```python
from build123d import *

# Parameters (mm, degrees)
SKETCH1_R           = 12.8
BOSS_EXTRUDE1_DEPTH = 23
SKETCH2_R           = 2
CUT_EXTRUDE1_DEPTH  = 7.5


with BuildPart() as part:
    # Sketch1 → Boss-Extrude1 (new, symmetric)
    with BuildSketch(Plane.XY):
        with BuildLine():
            Line((-13, -21.319), (13, -21.319))
            ThreePointArc((13, -21.319), (15.121320344, -20.440320344), (16, -18.319))
            Line((16, -18.319), (16, 12.7))
            ThreePointArc((16, 12.7), (15.121320344, 14.821320344), (13, 15.7))
            Line((13, 15.7), (-13, 15.7))
            ThreePointArc((-13, 15.7), (-15.121320344, 14.821320344), (-16, 12.7))
            Line((-16, 12.7), (-16, -18.319))
            ThreePointArc((-16, -18.319), (-15.121320344, -20.440320344), (-13, -21.319))
        make_face()
        Circle(SKETCH1_R, mode=Mode.SUBTRACT)
    extrude(amount=BOSS_EXTRUDE1_DEPTH, both=True)

    # Sketch2 → Cut-Extrude1 (cut)
    with BuildSketch(Plane(origin=(0, -21.319, 0), x_dir=(1, 0, 0), z_dir=(0, 1, 0))):
        with Locations(Location((12, -17.5, 0), (0, 0, 60))):
            Circle(SKETCH2_R)
        with Locations(Location((-12, 17.5, 0), (0, 0, 120))):
            Circle(SKETCH2_R)
    extrude(amount=CUT_EXTRUDE1_DEPTH, mode=Mode.SUBTRACT)


solid = part.part
```
The model under review builds one solid part; all positions refer to its coordinate system, in mm. A direction names the side the tool comes from. Give positions to 0.01 mm unless a question says otherwise; leave off trailing zeros. Write each loop counter-clockwise with the first axis right and the second up, starting at its lowest first coordinate (ties: lowest second). Pieces come first, ordered by that corner, then holes.
(1) Consider section B-B, the plane y = 0. Give the boundary of the cut face in (x, z), and give its area (3 significant figures).
(2) Consider section C-C, the plane z = 13.5. Give the boundary of the cut face in (x, y).
(3) Consider section D-D, the plane x = -12. Give the boundary of the cut face in (y, z).
(4) For P1, Ø1.2, axis at x = -12, z = -16.5, coming from the -Y side, flat-tipped, find the tip position at first contact; note if it passes through.
(5) To check wall thickness, follow L1, parallel to X at y = -17.25, z = 17.5; L2, parallel to Z at x = 12, y = -18.5; L3, parallel to X at y = -15.75, z = -17.5. State the ranges of each line that lie inside material, in increasing order.
(6) The part is to be moulded in two halves that separate along Y. For faces 1 (the cylindrical face through (-10.158, -7.789, -0.322)), 2 (the cylindrical face through (-15.1, 14.84, 0.32)), 3 (the flat face through (-7, -11, -23)), say which applies: released by +Y, released by -Y, zero draft, split by the parting line, or undercut.
(7) Tool access review of faces 4 (the cylindrical face through (-12.26, -17.622, -19.483)), 5 (the flat face through (0, -21.319, 0)): name each direction out of +Z, -Z, +X, -X, +Y, -Y from which nothing blocks a thin tool from reaching the whole face with its end or side.
(8) Consider section A-A, the plane x = 0. Give the boundary of the cut face in (y, z).
Returned:
1. outline: (-16, -23) - (-12.8, -23) - (-12.8, 23) - (-16, 23) - close; (12.8, -23) - (16, -23) - (16, 23) - (12.8, 23) - close
1. area: 294 mm2
2. outline: (-16, -18.32) arc R3 ccw to (-13, -21.32) - (13, -21.32) arc R3 ccw to (16, -18.32) - (16, 12.7) arc R3 ccw to (13, 15.7) - (-13, 15.7) arc R3 ccw to (-16, 12.7) - close; hole circle Ø25.6 at (0, 0)
3. outline: (-21.32, -23) - (-4.45, -23) - (-4.45, 23) - (-21.32, 23) - (-21.32, -15.5) - (-13.82, -15.5) - (-13.82, -19.5) - (-21.32, -19.5) - close; (4.45, -23) - (15.7, -23) - (15.7, 23) - (4.45, 23) - close
4. P1: stops at y = -13.82
5. L1: x = -16 to 10, 14 to 16
5. L2: z = -23 to 15.5, 19.5 to 23
5. L3: x = -16 to -14, -10 to 16
6. face 1: undercut
6. face 2: released by +Y
6. face 3: zero draft
7. face 4: -Y
7. face 5: +Z, -Z, +X, -X, -Y
8. outline: (-21.32, -23) - (-12.8, -23) - (-12.8, 23) - (-21.32, 23) - close; (12.8, -23) - (15.7, -23) - (15.7, 23) - (12.8, 23) - close
